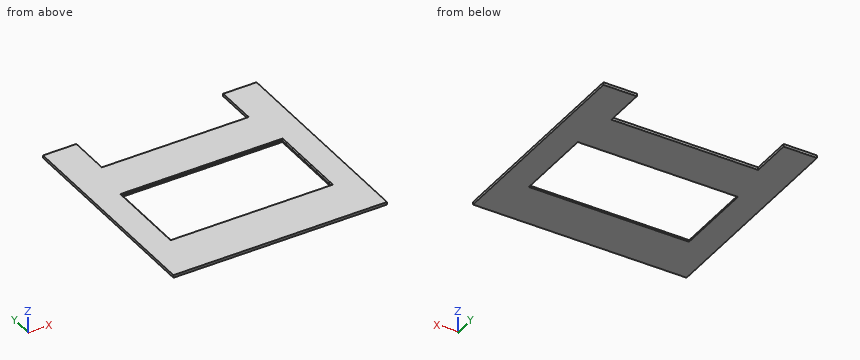
```python
from build123d import *

# Parameters (mm, degrees)
ESQUISSE1_W             = 400
ESQUISSE1_H             = 400
BOSS_EXTRU_1_DEPTH      = 5
ESQUISSE2_W             = 300
ESQUISSE2_H             = 150.02
ENL_V_MAT_EXTRU_1_DEPTH = 10
CHANFREIN1_SIZE         = 2
ESQUISSE3_W             = 275
ESQUISSE3_H             = 78.068424488
ENL_V_MAT_EXTRU_2_DEPTH = 283.886903196


with BuildPart() as part:
    # Esquisse1 → Boss.-Extru.1 (new body)
    with BuildSketch(Plane.XY):
        Rectangle(ESQUISSE1_W, ESQUISSE1_H)
    extrude(amount=BOSS_EXTRU_1_DEPTH)

    # Esquisse2 → Enlèv. mat.-Extru.1 (cut)
    with BuildSketch(Plane.XY.offset(5)):
        with Locations((0, -35.58)):
            Rectangle(ESQUISSE2_W, ESQUISSE2_H)
    extrude(amount=-ENL_V_MAT_EXTRU_1_DEPTH, mode=Mode.SUBTRACT)

    # Chanfrein1
    chanfrein1_edges = [part.edges().sort_by_distance(p)[0] for p in [
        (150, -35.58, 5),
        (0, 39.43, 5),
        (-150, -35.58, 5),
        (0, -110.59, 5),
    ]]
    chamfer(chanfrein1_edges, length=CHANFREIN1_SIZE)

    # Esquisse3 → Enlèv. mat.-Extru.2 (cut, through all)
    with BuildSketch(Plane.XY.offset(5)):
        with Locations((0, 160.965787756)):
            Rectangle(ESQUISSE3_W, ESQUISSE3_H)
    extrude(amount=-ENL_V_MAT_EXTRU_2_DEPTH, mode=Mode.SUBTRACT)


solid = part.part
```
Input: part model. Units: mm. Frame: model coordinates. Coordinates: 2 decimals unless noted, no trailing zeros. Loops run counter-clockwise (first coordinate to the right, second up) from the corner with the lowest first, then second, coordinate; pieces in that order, holes last. Notation, with made-up numbers: (-36.75, 6.5) - (-0.75, 6.5) arc R12 cw to (-0.75, 16.5) - close; hole circle Ø9 at (30, -26). An arc over 180 degrees is marked (long way). Answer in a Markdown table with one row per item.
(1) Material intervals for L1, parallel to Y at x = 40, z = 2.3; L2, parallel to X at y = -97.5, z = 1.95; L3, parallel to X at y = 177, z = 2.8, sorted ascending. Write a range as from..to.
Model answer:
| item | result |
|---|---|
| L1 | y = -200..-110.59, 39.43..121.93 |
| L2 | x = -200..-150, 150..200 |
| L3 | x = -200..-137.5, 137.5..200 |
(2) Cut plane B-B on y = -82. Output: boundary loops of the cut face in (x, z).
Model answer:
| item | result |
|---|---|
| outline | (-200, 0) - (-150, 0) - (-150, 3) - (-152, 5) - (-200, 5) - close; (150, 0) - (200, 0) - (200, 5) - (152, 5) - (150, 3) - close |
(3) Cut plane C-C on z = 0.8. Output: boundary loops of the cut face in (x, y), plus the area to 3 significant figures.
Model answer:
| item | result |
|---|---|
| outline | (-200, -200) - (200, -200) - (200, 200) - (137.5, 200) - (137.5, 121.93) - (-137.5, 121.93) - (-137.5, 200) - (-200, 200) - close; hole (-150, -110.59) - (150, -110.59) - (150, 39.43) - (-150, 39.43) - close |
| area | 93,500 mm² |
(4) Cut plane A-A on x = 99. Output: boundary loops of the cut face in (y, z), plus the area to 3 significant figures.
Model answer:
| item | result |
|---|---|
| outline | (-200, 0) - (-110.59, 0) - (-110.59, 3) - (-112.59, 5) - (-200, 5) - close; (39.43, 0) - (121.93, 0) - (121.93, 5) - (41.43, 5) - (39.43, 3) - close |
| area | 856 mm² |
